Verification items for the finished model (mm, model axes). Face numbers are marked on the shaded views. Give positions to 0.01 mm unless a question says otherwise; leave off trailing zeros. Use one line per item in the form item = value.
```python
from build123d import *

# Parameters (mm, degrees)
F1_DEPTH = 15.875
F2_R     = 3.175
F3_DEPTH = 50.8
F4_R     = 3.175
F5_DEPTH = 25.4
F6_SIZE  = 1.905


with BuildPart() as f1:
    # F0 (on Top) → F1 (new body)
    with BuildSketch(Plane.XY):
        with BuildLine():
            ThreePointArc((-55.540178, 1.5748), (55.562499, 0.012705), (-55.539452, -1.6002))
            Line((-55.539452, -1.6002), (-93.413361, -1.6002))
            Line((-93.413361, -1.6002), (-93.413361, -71.873484))
            Line((-93.413361, -71.873484), (65.0875, -71.873484))
            Line((65.0875, -71.873484), (65.0875, 0))
            ThreePointArc((65.0875, 0), (22.536226, 61.061454), (-49.481386, 42.284454))
            ThreePointArc((-49.481386, 42.284454), (-53.820886, 39.000936), (-59.136291, 37.835079))
            Line((-59.136291, 37.835079), (-83.994267, 37.835079))
            ThreePointArc((-83.994267, 37.835079), (-90.208527, 35.528708), (-93.413361, 29.726516))
            Line((-93.413361, 29.726516), (-93.413361, 26.893643))
            Line((-93.413361, 26.893643), (-93.413361, 1.5748))
            Line((-93.413361, 1.5748), (-55.540178, 1.5748))
        make_face()
        with BuildLine():
            ThreePointArc((-93.413361, 29.726516), (-93.519267, 28.310079), (-93.413361, 26.893643))
            Line((-93.413361, 26.893643), (-93.413361, 29.726516))
        make_face()
    extrude(amount=F1_DEPTH)

    # F2 (on face) → F3 (cut)
    with BuildSketch(Plane(origin=(0, 37.835079, 0), x_dir=(-1, 0, 0), z_dir=(0, 1, 0))):
        with Locations((76.069467, 7.9502)):
            Circle(F2_R)
    extrude(amount=-F3_DEPTH, mode=Mode.SUBTRACT)

    # F4 (on face) → F5 (cut)
    with BuildSketch(Plane.XZ.offset(71.873484)):
        with Locations((-38.1, 7.9375)):
            Circle(F4_R)
        with Locations((38.1, 7.9375)):
            Circle(F4_R)
    extrude(amount=-F5_DEPTH, mode=Mode.SUBTRACT)

    # F6
    f6_edges = [f1.edges().sort_by_distance(p)[0] for p in [
        (55.562499, 0.012705, 15.875),
        (-74.476406, -1.6002, 15.875),
        (-93.413361, -36.736842, 15.875),
        (-14.16293, -71.873484, 15.875),
        (65.0875, -35.936742, 15.875),
        (22.536226, 61.061454, 15.875),
        (-53.820886, 39.000936, 15.875),
        (-71.565279, 37.835079, 15.875),
        (-91.212895, 34.52434, 15.875),
        (-93.413361, 14.234221, 15.875),
        (-74.476769, 1.5748, 15.875),
        (55.562499, 0.012705, 0),
        (-74.476406, -1.6002, 0),
        (-93.413361, -36.736842, 0),
        (-14.16293, -71.873484, 0),
        (65.0875, -35.936742, 0),
        (22.536226, 61.061454, 0),
        (-53.820886, 39.000936, 0),
        (-71.565279, 37.835079, 0),
        (-91.212895, 34.52434, 0),
        (-93.413361, 14.234221, 0),
        (-74.476769, 1.5748, 0),
    ]]
    chamfer(f6_edges, length=F6_SIZE)


solid = f1.part
```
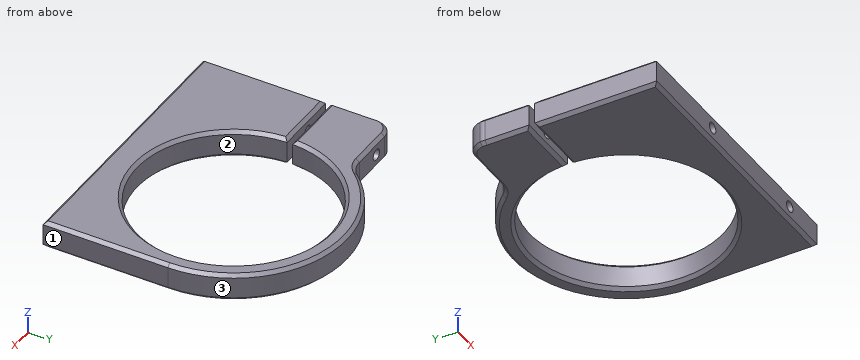
1. Draft check along Y on the marked faces 1, 2 and 3. Enter one of: released by +Y, released by -Y, zero draft, split by the parting line, or undercut.
Result set:
face_1 = zero draft
face_2 = undercut
face_3 = released by +Y
2. Scan lines: probe 1 along X at (y, z) = (-58.5, 8.25); probe 2 along Y at (x, z) = (0, 6); probe 3 along X at (y, z) = (20, 6.25). Record each from-to range of solid material in increasing order.
Result set:
probe_1 = -93.41 to -41.26, -34.94 to 34.94, 41.26 to 65.09
probe_2 = -71.87 to -55.56, 55.56 to 65.09
probe_3 = -93.41 to -78.75, -73.39 to -51.84, 51.84 to 61.94
3. Depth check by flat-ended pin: pin 1 Ø5 at (x, z) = (-76.07, 7.95) entering from +Y; pin 2 Ø3.5 at (x, z) = (-80.5, 6.5) entering from +Y; pin 3 Ø5 at (x, z) = (-38.1, 7.94) entering from +Y. Enter the tip coordinate at first touch or a pass-through.
Result set:
pin_1 = -12.96
pin_2 = 37.84
pin_3 = 54.49
4. Section check A-A, the plane y = -62. State how many separate pieces and enclosed holes the cut face has, then the cut area to 3 significant figures.
Result set:
separate_pieces = 1
enclosed_holes = 2
area = 2,450 mm²
